from build123d import *

# Parameters (mm, degrees)
SKETCH1_R               = 113.538
BOSS_EXTRUDE1_DEPTH     = 84.836
CUT_EXTRUDE1_DEPTH      = 182.600941033
CUT_EXTRUDE1_DEPTH_BACK = 182.600941033
SKETCH2_R               = 4.445
SKETCH4_R               = 23.841151021
BOSS_EXTRUDE2_DEPTH     = 13.97


with BuildPart() as part:
    # Sketch1 → Boss-Extrude1 (new body)
    with BuildSketch(Plane.XY):
        Circle(SKETCH1_R)
    extrude(amount=-BOSS_EXTRUDE1_DEPTH)

    # Sketch2 → Cut-Extrude1 (cut, two sides: drawn at the far end of the back side and taken through both)
    with BuildSketch(Plane.XY.offset(-CUT_EXTRUDE1_DEPTH_BACK)):
        with Locations((0, 37.49999993)):
            Circle(SKETCH2_R)
        with Locations((32.475952581, 18.749999965)):
            Circle(SKETCH2_R)
        with Locations((32.475952581, -18.749999965)):
            Circle(SKETCH2_R)
        with Locations((0, -37.49999993)):
            Circle(SKETCH2_R)
        with Locations((-32.475952581, -18.749999965)):
            Circle(SKETCH2_R)
        with Locations((-32.475952581, 18.749999965)):
            Circle(SKETCH2_R)
    extrude(amount=CUT_EXTRUDE1_DEPTH + CUT_EXTRUDE1_DEPTH_BACK, mode=Mode.SUBTRACT)

    # Sketch4 → Boss-Extrude2 (add)
    with BuildSketch(Plane(origin=(0, 0, -84.836), x_dir=(-1, 0, 0), z_dir=(0, 0, -1))):
        with Locations(Location((0, 0, 0), (0, 0, 180))):
            Circle(SKETCH4_R)
    extrude(amount=BOSS_EXTRUDE2_DEPTH)


solid = part.part
Geometry: final body of the model. Coordinates: model frame, mm. A direction names the side the tool comes from. Coordinates: 2 decimals unless noted, no trailing zeros. Order: outer loops, then holes, each group sorted by start corner. A loop starts at its lowest first (then second) coordinate and runs counter-clockwise, first axis right, second up.
(1) Section query A-A (x = 0). Return the cut outline in (y, z) (3 decimals).
(2) Draft query along X for faces 1 (the face through (2.051, 33.557, -43.012)), 2 (the face through (-24.61, -110.84, -41.82)), 3 (the face through (-2, 2, 0)). Return one class per face: pulls with the +X half, pulls with the -X half, needs draft (parallel to the pull), parting line crosses it, or undercut.
(3) Access query for faces 4 (the face through (11, 21.15, -91.72)), 5 (the face through (-28.236, 20.085, -43.012)). Directions: +Z, -Z, +X, -X, +Y, -Y. A direction counts if a zero-diameter tool reaches every point of the face in a straight line with its end or side. Return the directions, or none.
(4) First-contact query: pin 1 (1 mm diameter, centred on y = 61.5, z = -16.5, fed in from +X); pin 2 (8 mm diameter, centred on x = -53, y = -72.5, fed in from +Z); pin 3 (1.5 mm diameter, centred on y = 76.5, z = -67, fed in from +X); pin 4 (5 mm diameter, centred on x = -47.5, y = 47, fed in from -Z). Flat tips, straight axial feed; report the tip coordinate or a pass-through.
(5) Section query C-C (y = 0). Return the cut outline in (x, z), plus the area to 3 significant figures.
(6) Section query D-D (y = 37.5). Return the cut outline in (x, z) (3 decimals).
(7) Section query B-B (z = -36.5). Return the cut outline in (x, y) (3 decimals), plus the area to 3 significant figures.
(8) Material intervals for probe 1 along Y at (x, z) = (0, -36) (3 decimals); probe 2 along X at (y, z) = (18.75, -49.5); probe 3 along Z at (x, y) = (-13, -43), sorted ascending.
Solution:
1. outline: (-113.538, -84.836) - (-41.945, -84.836) - (-41.945, 0) - (-113.538, 0) - close; (-33.055, -84.836) - (-23.841, -84.836) - (-23.841, -98.806) - (23.841, -98.806) - (23.841, -84.836) - (33.055, -84.836) - (33.055, 0) - (-33.055, 0) - close; (41.945, -84.836) - (113.538, -84.836) - (113.538, 0) - (41.945, 0) - close
2. face 1: undercut
2. face 2: parting line crosses it
2. face 3: needs draft
3. face 4: -Z
3. face 5: +Z, -Z
4. pin 1: stops at x = 95.76
4. pin 2: stops at z = 0
4. pin 3: stops at x = 84.57
4. pin 4: stops at z = -84.84
5. outline: (-113.54, -84.84) - (-23.84, -84.84) - (-23.84, -98.81) - (23.84, -98.81) - (23.84, -84.84) - (113.54, -84.84) - (113.54, 0) - (-113.54, 0) - close
5. area: 19,900 mm2
6. outline: (-107.166, -84.836) - (-4.445, -84.836) - (-4.445, 0) - (-107.166, 0) - close; (4.445, -84.836) - (107.166, -84.836) - (107.166, 0) - (4.445, 0) - close
7. outline: circle Ø227.076 at (0, 0); hole circle Ø8.89 at (-32.476, -18.75); hole circle Ø8.89 at (-32.476, 18.75); hole circle Ø8.89 at (0, -37.5); hole circle Ø8.89 at (0, 37.5); hole circle Ø8.89 at (32.476, -18.75); hole circle Ø8.89 at (32.476, 18.75)
7. area: 40,100 mm2
8. probe 1: y = -113.538 to -41.945, -33.055 to 33.055, 41.945 to 113.538
8. probe 2: x = -111.98 to -36.92, -28.03 to 28.03, 36.92 to 111.98
8. probe 3: z = -84.84 to 0
